```python
from build123d import *

# Parameters (mm, degrees)
SKETCH_1_R         = 3.25
EXTRUDE_1058_DEPTH = 3
FILLET_1_R         = 10
HOLE_WIZARD_3_2_D  = 3.5


with BuildPart() as part:
    # Эскиз1 → Extrude 1058 (new, symmetric)
    with BuildSketch(Plane(origin=(0, 0, 0), x_dir=(1, 0, 0), z_dir=(0, 1, 0))):
        Polygon((273.664027596, -136.63804004), (18.5, 305.31902002), (-18.5, 305.31902002), (-273.664027596, -136.63804004), (-255.164027596, -168.68097998), (255.164027596, -168.68097998), align=None)
        with Locations(Location((0, 289.31902002, 0), (0, 0, 270))):
            Circle(SKETCH_1_R, mode=Mode.SUBTRACT)
        with Locations(Location((-250.557621135, -144.65951001, 0), (0, 0, 270))):
            Circle(SKETCH_1_R, mode=Mode.SUBTRACT)
        with Locations(Location((250.557621135, -144.65951001, 0), (0, 0, 270))):
            Circle(SKETCH_1_R, mode=Mode.SUBTRACT)
    extrude(amount=EXTRUDE_1058_DEPTH, both=True)

    # Скругление1
    fillet_1_edges = [part.edges().sort_by_distance(p)[0] for p in [
        (255.164027596, 0, 168.68097998),
        (-255.164027596, 0, 168.68097998),
        (-273.664027596, 0, 136.63804004),
        (-18.5, 0, -305.31902002),
        (18.5, 0, -305.31902002),
        (273.664027596, 0, 136.63804004),
    ]]
    fillet(fillet_1_edges, radius=FILLET_1_R)

    # К Профилю 3,2мм (through all)
    with Locations(Plane(origin=(0, -3, 0), x_dir=(-1, 0, 0), z_dir=(0, -1, 0))):
        with Locations((150, -158.68097998), (0, -158.68097998), (-150, -158.68097998), (-212.42175976, -50.563320578), (-137.42175976, 79.34048999), (-62.42175976, 209.244300558), (62.42175976, 209.244300558), (137.42175976, 79.34048999), (212.42175976, -50.563320578)):
            Hole(HOLE_WIZARD_3_2_D / 2)


solid = part.part
```
Geometry check sheet. Reference: the model listing, model coordinates, mm. Coordinates: 2 decimals unless noted, no trailing zeros. Write each loop counter-clockwise with the first axis right and the second up, starting at its lowest first coordinate (ties: lowest second). Pieces come first, ordered by that corner, then holes. Notation, with made-up numbers: M -29.75,-29 L -6.75,-29 A19 ccw -6.75,-12 Z; hole C 11,37.5 d3. An arc over 180 degrees is marked long. One line per item, written item: value. Start each with the question number.
(1) Sectioned sample at B-B, the plane z = -123. Enter the section's corners in (x, y), and give its area (3 significant figures).
(2) Depth check by flat-ended pin: pin 1 (5.5 mm diameter, centred on x = -150, z = 158.68, fed in from -Y); pin 2 (3 mm diameter, centred on x = 137.42, z = -79.34, fed in from +Y); pin 3 (1 mm diameter, centred on x = 28.5, y = 2, fed in from -Z); pin 4 (2 mm diameter, centred on y = -2, z = -50.5, fed in from +X). Enter the tip coordinate at first touch or a pass-through.
(3) Sectioned sample at A-A, the plane y = -1.95. State how many separate pieces and enclosed holes the cut face has, and give its area (3 significant figures).
(4) Sectioned sample at C-C, the plane x = -231.5. Enter the section's corners in (y, z), and give its area (3 significant figures).
(5) Scan lines: line 1 along Z through (x, y) = (150, 1.4); line 2 along Z through (x, y) = (-223, 1.5); line 3 along X through (y, z) = (2.8, 42.5). Record each from-to range of solid material in increasing order. Write a range as [from, to].
Filled sheet:
1. outline: M -123.76,-3 L 123.76,-3 L 123.76,3 L -123.76,3 Z
1. area: 1,490 mm²
2. pin 1: y = -3
2. pin 2: through
2. pin 3: z = -288.86
2. pin 4: x = 166.2
3. separate pieces: 1
3. enclosed holes: 12
3. area: 146,000 mm²
4. outline: M -3,63.61 L 3,63.61 L 3,168.68 L -3,168.68 Z
4. area: 630 mm²
5. line 1: [-77.55, 156.93], [160.43, 168.68]
5. line 2: [48.89, 168.68]
5. line 3: [-219.31, 219.31]
